Design review of the part built by this model. Coordinates are the model's own, in mm. Coordinates: 2 decimals unless noted, no trailing zeros. Write each loop counter-clockwise with the first axis right and the second up, starting at its lowest first coordinate (ties: lowest second). Pieces come first, ordered by that corner, then holes.
Q1. Take a section at A-A, the plane y = -132.5. Write out the cut boundary in (x, z), plus the area to 3 significant figures.
Q2. For L1, parallel to Z at x = 0, y = -163.6; L2, parallel to Y at x = 0.5, z = 0.5; L3, parallel to Z at x = 0.25, y = 36, list the stretches that pass through material, from the lowest coordinate up.
Q3. For pin 1 Ø3.5 at (x, z) = (-0.5, 0) entering from +Y; pin 2 Ø2 at (x, y) = (-3, -104) entering from +Z; pin 3 Ø1.5 at (x, z) = (-0.5, 0.5) entering from -Y, all flat-tipped, find the tip position at first contact; note any pin that passes through.
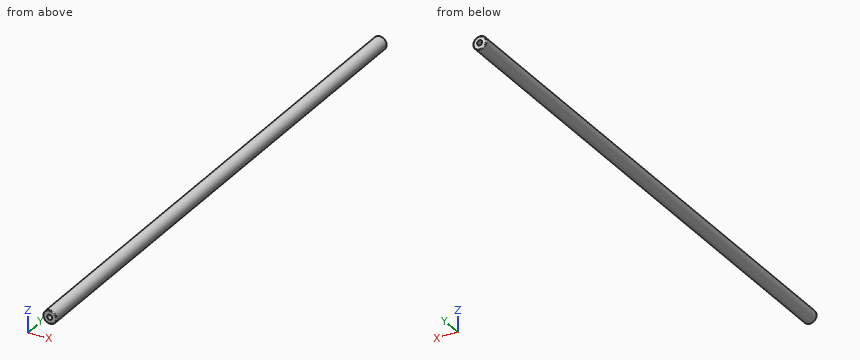
Autodesk Inventor part; units mm, degrees
ref_plane "YZ Plane" through (0, 0, 0) normal (1, 0, 0) x (0, 1, 0)
ref_plane "XZ Plane" through (0, 0, 0) normal (0, 1, 0) x (-1, 0, 0)
ref_plane "XY Plane" through (0, 0, 0) normal (0, 0, 1) x (1, 0, 0)
sketch "Эскиз1" plane through (0, 0, 0) normal (0, 1, 0) x (-1, 0, 0)
  circle A0 centre (0, 0) radius 4
  dimension "d0" = 8
extrude "Выдавливание1" add sketch "Эскиз1" along normal mid plane 329.9
sketch "Эскиз2" plane through (0, 164.95, 0) normal (0, 1, 0) x (1, 0, 0)
  circle A0 centre (0, 0) radius 1.5
  dimension "d3" = 3
extrude "Выдавливание2" cut sketch "Эскиз2" against normal blind 5
mirror "Зеркальное отражение1" about plane through (0, 0, 0) normal (0, 1, 0) of "Выдавливание2"
fillet "Сопряжение1" radius 0.5 2 edges at (4, -164.95, 0) (4, 164.95, 0)
properties part number "вал 8мм"
Responses:
1. outline: circle Ø8 at (0, 0)
1. area: 50.3 mm2
2. L1: z = -4 to -1.5, 1.5 to 4
2. L2: y = -159.95 to 159.95
2. L3: z = -3.99 to 3.99
3. pin 1: stops at y = 164.95
3. pin 2: stops at z = 3.46
3. pin 3: stops at y = -159.95
